For this review, use the dimensioned drawing (mm, ordinates from the lowest corner) and the shaded views. A direction names the side the tool comes from. Coordinates: 2 decimals unless noted, no trailing zeros. Order: outer loops, then holes, each group sorted by start corner. A loop starts at its lowest first (then second) coordinate and runs counter-clockwise, first axis right, second up. Notation, with made-up numbers: M 67.25,15.25 L 97.25,15.25 A31 ccw 97.25,53.25 Z; hole C 1,44 d2. An arc over 180 degrees is marked long. Answer as CSV lines item,"result". Start each with the question number.
Q1. Consider section D-D on y = 35. Write out the cut boundary in (x, z), and give its area (3 significant figures).
Q2. Consider section C-C on x = 12. Write out the cut boundary in (y, z), and give its area (3 significant figures).
Q3. Consider section B-B on y = 25. Write out the cut boundary in (x, z), and give its area (3 significant figures).
Q4. Wall thickness on L1, parallel to Y at x = 20, z = 1.4; L2, parallel to Z at x = 17, y = 37.5; L3, parallel to Y at x = 63, z = 11.75: over which ranges is each line inside the solid? List them lowest first. Write a range as [from, to].
Q5. Machinability: for the marked faces 1 and 2, which of the approach directions +Z, -Z, +X, -X, +Y, -Y give a long, thin tool a straight path to every point of the face, cutting with its end or side? Answer none if there is none.
Q6. For P1, Ø4, axis at x = 82, z = 7.5, coming from the +Y side; P2, Ø5, axis at x = 70, y = 6.5, coming from the +Z side; P3, Ø2, axis at x = 38.5, z = 8.5, coming from the -Y side, all flat-tipped, find the tip position at first contact; note any pin that passes through.
Q7. Consider section A-A on x = 78.5. Write out the cut boundary in (y, z), and give its area (3 significant figures).
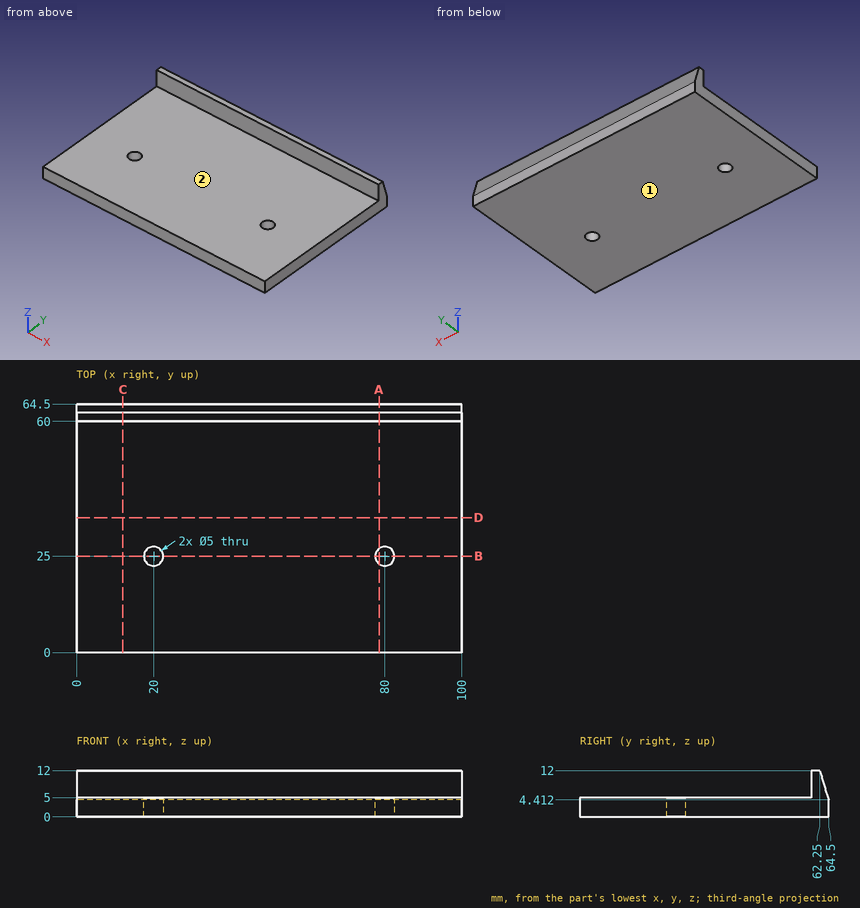
Evaluation:
1,outline,"M 0,0 L 100,0 L 100,5 L 0,5 Z"
1,area,"500 mm²"
2,outline,"M 0,0 L 64.5,0 L 64.5,4.41 L 62.25,12 L 60,12 L 60,5 L 0,5 Z"
2,area,"345 mm²"
3,outline,"M 0,0 L 17.5,0 L 17.5,5 L 0,5 Z; M 22.5,0 L 77.5,0 L 77.5,5 L 22.5,5 Z; M 82.5,0 L 100,0 L 100,5 L 82.5,5 Z"
3,area,"450 mm²"
4,L1,"y = [0, 22.5], [27.5, 64.5]"
4,L2,"z = [0, 5]"
4,L3,"y = [60, 62.32]"
5,face 1,"-Z, +X, -X, +Y, -Y"
5,face 2,"+Z, +X, -X, -Y"
6,P1,"stops at y = 64.18"
6,P2,"stops at z = 5"
6,P3,"stops at y = 60"
7,outline,"M 0,0 L 23,0 L 23,5 L 0,5 Z; M 27,0 L 64.5,0 L 64.5,4.41 L 62.25,12 L 60,12 L 60,5 L 27,5 Z"
7,area,"325 mm²"
